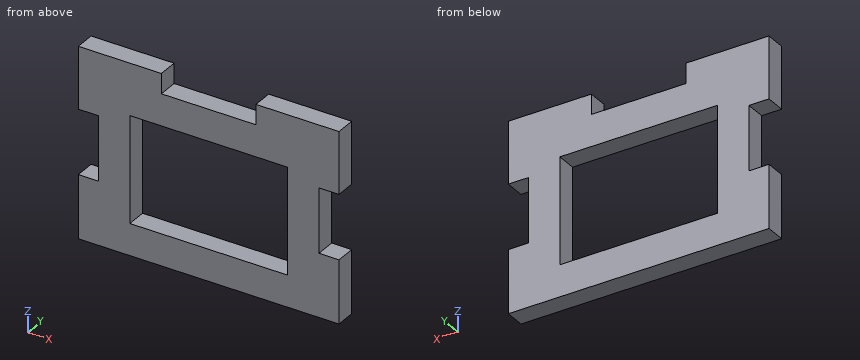
from build123d import *

# Parameters (mm, degrees)
SKETCH1_W               = 41.35
SKETCH1_H               = 30
BOSS_EXTRUDE1_DEPTH     = 3.175
SKETCH2_W               = 3.175
SKETCH2_H               = 10.2
SKETCH2_W_2             = 15
SKETCH2_H_2             = 3.175
CUT_EXTRUDE1_DEPTH      = 4.175
SKETCH3_W               = 25
SKETCH3_H               = 16.825
CUT_EXTRUDE2_DEPTH      = 1
CUT_EXTRUDE2_DEPTH_BACK = 4.175


with BuildPart() as part:
    # Sketch1 → Boss-Extrude1 (new body)
    with BuildSketch(Plane(origin=(0, 0, 0), x_dir=(1, 0, 0), z_dir=(0, 1, 0))):
        with Locations((20.675, 15)):
            Rectangle(SKETCH1_W, SKETCH1_H)
    extrude(amount=BOSS_EXTRUDE1_DEPTH)

    # Sketch2 → Cut-Extrude1 (cut, through all)
    with BuildSketch(Plane.XZ):
        with Locations((1.5875, -14.9)):
            Rectangle(SKETCH2_W, SKETCH2_H)
        with Locations((39.7625, -14.9)):
            Rectangle(SKETCH2_W, SKETCH2_H)
        with Locations((20.675, -1.5875)):
            Rectangle(SKETCH2_W_2, SKETCH2_H_2)
    extrude(amount=-CUT_EXTRUDE1_DEPTH, mode=Mode.SUBTRACT)

    # Sketch3 → Cut-Extrude2 (cut, two sides)
    with BuildSketch(Plane(origin=(0, 3.175, 0), x_dir=(1, 0, 0), z_dir=(0, 1, 0))) as cut_extrude2_sk:
        with Locations((20.675, 16.5875)):
            Rectangle(SKETCH3_W, SKETCH3_H)
    extrude(amount=CUT_EXTRUDE2_DEPTH, mode=Mode.SUBTRACT)
    extrude(cut_extrude2_sk.sketch, amount=-CUT_EXTRUDE2_DEPTH_BACK, mode=Mode.SUBTRACT)


solid = part.part
Could you check a few things on this model? Use its own coordinates, in mm. Give positions to 0.01 mm unless a question says otherwise; leave off trailing zeros. Order: outer loops, then holes, each group sorted by start corner. A loop starts at its lowest first (then second) coordinate and runs counter-clockwise, first axis right, second up. Notation, with made-up numbers: (18.5, 2) -> (33.5, 2) arc R18 cw to (33.5, 11) -> close; hole circle Ø2 at (29.25, 63). An arc over 180 degrees is marked (long way). Answer in a Markdown table with one row per item. Add a question column.
Item 1: Imagine slicing it at B-B (x = 32). List the corners of the cut face in (y, z) for me (3 decimals).
Item 2: Imagine slicing it at A-A (z = -19). List the corners of the cut face in (x, y) for me (3 decimals), and give its area (4 significant figures).
Item 3: Please list where these lines run through material, in increasing order: probe 1 along X at (y, z) = (0.45, -2.75) (3 decimals); probe 2 along X at (y, z) = (1.4, -15) (3 decimals); probe 3 along Z at (x, y) = (11, 2.15) (3 decimals).
Item 4: Imagine slicing it at C-C (y = 1.8). List the corners of the cut face in (x, z) for me (3 decimals), and give its area (3 significant figures).
Result:
| question | item | result |
|---|---|---|
| 1 | outline | (0, -30) -> (3.175, -30) -> (3.175, -25) -> (0, -25) -> close; (0, -8.175) -> (3.175, -8.175) -> (3.175, 0) -> (0, 0) -> close |
| 2 | outline | (3.175, 0) -> (8.175, 0) -> (8.175, 3.175) -> (3.175, 3.175) -> close; (33.175, 0) -> (38.175, 0) -> (38.175, 3.175) -> (33.175, 3.175) -> close |
| 2 | area | 31.75 mm2 |
| 3 | probe 1 | 0 to 13.175, 28.175 to 41.35 |
| 3 | probe 2 | 3.175 to 8.175, 33.175 to 38.175 |
| 3 | probe 3 | -30 to -25, -8.175 to 0 |
| 4 | outline | (0, -30) -> (41.35, -30) -> (41.35, -20) -> (38.175, -20) -> (38.175, -9.8) -> (41.35, -9.8) -> (41.35, 0) -> (28.175, 0) -> (28.175, -3.175) -> (13.175, -3.175) -> (13.175, 0) -> (0, 0) -> (0, -9.8) -> (3.175, -9.8) -> (3.175, -20) -> (0, -20) -> close; hole (8.175, -25) -> (33.175, -25) -> (33.175, -8.175) -> (8.175, -8.175) -> close |
| 4 | area | 707 mm2 |
